from build123d import *

# Parameters (mm, degrees)
SKETCH1_W                    = 50
SKETCH1_H                    = 40
BASE_FLANGE1_DEPTH           = 2
EDGE_FLANGE1_STRIP_W         = 9.4732
EDGE_FLANGE1_STRIP_H         = 2
EDGE_FLANGE1_STRIP_CUT_DEPTH = 50
EDGE_FLANGE1_DEPTH           = 50
ADVANCEDHOLE2_START          = -17.684659091
ADVANCEDHOLE2_OUTLINE_R      = 3
ADVANCEDHOLE2_DEPTH          = 2


# Read off the part's stored shape, not the designer's step: AdvancedHole2
# Sheet-metal steps are written as plain solids
with BuildPart() as part:
    # Sketch1 → Base-Flange1 (new body)
    with BuildSketch(Plane(origin=(0, 0, 0), x_dir=(1, 0, 0), z_dir=(0, 1, 0))):
        with Locations((-3.551136364, -2.315340909)):
            Rectangle(SKETCH1_W, SKETCH1_H)
    extrude(amount=-BASE_FLANGE1_DEPTH)

    # Edge-Flange1 strip (across the edge) → Edge-Flange1 strip cut (cut)
    with BuildSketch(Plane(origin=(21.448863636, 0, -17.684659091), x_dir=(0, 0, 1), z_dir=(-1, 0, 0))):
        with Locations((-2, -1)):
            Rectangle(EDGE_FLANGE1_STRIP_W, EDGE_FLANGE1_STRIP_H)
    extrude(amount=EDGE_FLANGE1_STRIP_CUT_DEPTH, mode=Mode.SUBTRACT)

    # Edge-Flange1 section (across the edge) → Edge-Flange1 (add)
    with BuildSketch(Plane(origin=(21.448863636, 0, -17.684659091), x_dir=(0, 0, 1), z_dir=(-1, 0, 0))):
        with BuildLine():
            Line((0, 0.7366), (0, 78))
            Line((0, 78), (2, 78))
            Line((2, 78), (2, 0.7366))
            ThreePointArc((2, 0.7366), (2.215745145, 0.215745145), (2.7366, 0))
            Line((2.7366, 0), (2.7366, -2))
            ThreePointArc((2.7366, -2), (0.801531583, -1.198468417), (0, 0.7366))
        make_face()
    extrude(amount=EDGE_FLANGE1_DEPTH)

    # AdvancedHole2 outline → AdvancedHole2 (cut)
    with BuildSketch(Plane.XY.offset(ADVANCEDHOLE2_START)):
        with Locations((-3.551136364, 54)):
            Circle(ADVANCEDHOLE2_OUTLINE_R)
    extrude(amount=ADVANCEDHOLE2_DEPTH, mode=Mode.SUBTRACT)


solid = part.part
Can you work these out from the model? Positions are in its coordinate system, mm. A direction names the side the tool comes from. Coordinates: 2 decimals unless noted, no trailing zeros. Order: outer loops, then holes, each group sorted by start corner. A loop starts at its lowest first (then second) coordinate and runs counter-clockwise, first axis right, second up. Notation, with made-up numbers: M 73.25,50 L 114.25,50 A28 cw 114.25,70 Z; hole C -18,72.5 d6. An arc over 180 degrees is marked long. Write item = value, one per line.
(1) For faces 5 (the face through (-3, 78, -17)), 6 (the face through (-3, 40, -15.685)), which set-ups out of +Z, -Z, +X, -X, +Y, -Y let a thin tool reach every point of the face, with its end or its side?
Results are:
face_5 = +Z, -Z, +X, -X, +Y
face_6 = +Z, +X, -X, +Y
(2) Suppose I cut it at D-D on z = 0.5. Please give me the cut outline in (x, y), plus the area to 3 significant figures.
Results are:
outline = M -28.55,-2 L 21.45,-2 L 21.45,0 L -28.55,0 Z
area = 100 mm2
(3) Suppose I cut it at A-A on y = 54. Please give me the cut outline in (x, z).
Results are:
outline = M -28.55,-17.68 L -6.55,-17.68 L -6.55,-15.68 L -28.55,-15.68 Z; M -0.55,-17.68 L 21.45,-17.68 L 21.45,-15.68 L -0.55,-15.68 Z
(4) Suppose I cut it at B-B on x = -23. Please give me the cut outline in (y, z), plus the area to 3 significant figures.
Results are:
outline = M -2,-14.95 A2.74 ccw 0.74,-17.68 L 78,-17.68 L 78,-15.68 L 0.74,-15.68 A0.74 cw 0,-14.95 L 0,22.32 L -2,22.32 Z
area = 235 mm2
(5) If we mould it in two halves opening along X, with no side actions, what happens to faces 1 (the face through (-28.551, 20, -17)), 2 (the face through (-4, -2, 3)), 3 (the face through (-3.942, 56.974, -16.699)), 4 (the face through (21.449, 20, -17))? For each: pulls with the +X half, pulls with the -X half, needs draft (parallel to the pull), parting line crosses it, or undercut.
Results are:
face_1 = pulls with the -X half
face_2 = needs draft
face_3 = undercut
face_4 = pulls with the +X half
(6) Suppose I cut it at C-C on x = -1.5. Please give me the cut outline in (y, z), plus the area to 3 significant figures.
Results are:
outline = M -2,-14.95 A2.74 ccw 0.74,-17.68 L 51.81,-17.68 L 51.81,-15.68 L 0.74,-15.68 A0.74 cw 0,-14.95 L 0,22.32 L -2,22.32 Z; M 56.19,-17.68 L 78,-17.68 L 78,-15.68 L 56.19,-15.68 Z
area = 226 mm2
(7) For pin 1 Ø2 at (x, z) = (-8.5, 13.5) entering from +Y; pin 2 Ø7 at (x, y) = (-3.55, 54) entering from +Z, each with a flat end and sliding along its axis, tell me the tip position at first contact or that it passes through.
Results are:
pin_1 = 0
pin_2 = -15.68
(8) I need wall thicknesses on line 1 along Y through (x, z) = (17, 1.5); line 2 along Z through (x, y) = (-25.5, 17.5). Which ranges of each line are inside material? Lowest first, please. Write a range as [from, to].
Results are:
line_1 = [-2, 0]
line_2 = [-17.68, -15.68]
